Part model, mm, in its own coordinate system. A direction names the side the tool comes from. Round coordinates to 2 decimals unless told otherwise and drop trailing zeros. Loops run counter-clockwise (first coordinate to the right, second up) from the corner with the lowest first, then second, coordinate; pieces in that order, holes last. Notation, with made-up numbers: M 22.25,40 L 30.25,40 A5 ccw 30.25,48 Z; hole C -14,-37.5 d11. An arc over 180 degrees is marked long. Answer as CSV lines item,"result". Start each with the question number.
Item 1: Band-saw the part on C-C (y = -1.5). Give the cut face in (x, z), and give its area (3 significant figures).
Item 2: Which spindle directions (+Z, -Z, +X, -X, +Y, -Y) get a long thin tool onto all of the face, cutting with end or side? Do faces 4 (the cylindrical face through (0, 8.5, 5.6)), 5 (the cylindrical face through (-4.66, -8.85, 5.42)), 6 (the flat face through (8.3, -2.7, 11)), 7 (the cylindrical face through (2.406, 9.706, 5.423)), 8 (the cylindrical face through (-9.346, 3.558, 5.423)). Say none if no direction does.
Item 3: Wall check: line 1 (Y direction, x = 0, z = 3.75); line 2 (Z direction, x = 10.5, y = -6.5); line 3 (Y direction, x = 9.25, z = 3.25). Give the ranges that are in metal, low to high.
Item 4: Drop flat-ended pins along their axis: pin 1 Ø8 at (y, z) = (-7, -0.5) entering from -X; pin 2 Ø5 at (y, z) = (8, 8) entering from -X; pin 3 Ø3 at (x, y) = (0, 0) entering from -Z; pin 4 Ø1.5 at (x, z) = (0.5, 11) entering from +Y. Give the stop position or say it passes through.
Item 5: Band-saw the part on B-B (z = 8.5). Give the cut face in (x, y).
Item 6: Band-saw the part on A-A (x = 0). Give the cut face in (y, z), and give its area (3 significant figures).
Item 7: Band-saw the part on D-D (y = 3.5). Give the cut face in (x, z).
Item 8: Mould opens along X. For faces 1 (the flat face through (0, -3, 13)), 2 (the cylindrical face through (-8, -6, 5)), 3 (the cylindrical face through (-5.613, -6.383, 5.577)) say: pulls with the +X half, pulls with the -X half, needs draft (parallel to the pull), parting line crosses it, or undercut.
```python
from build123d import *

# Parameters (mm, degrees)
F0_R     = 10
F1_DEPTH = 11
F2_R     = 1.5
F3_DEPTH = 25
F4_R     = 12.5
F5_DEPTH = 2
F6_R     = 12.5
F7_DEPTH = 2
F8_R     = 2.55
F9_DEPTH = 15.001


with BuildPart() as f1:
    # F0 (on Top) → F1 (new body)
    with BuildSketch(Plane.XY):
        Circle(F0_R)
    extrude(amount=F1_DEPTH)

    # F2 (on face) → F3 (cut)
    with BuildSketch(Plane.XY.offset(11)):
        with Locations((0, 10)):
            Circle(F2_R)
        with Locations((-4.647232, 8.85456)):
            Circle(F2_R)
        with Locations((-8.229839, 5.680647)):
            Circle(F2_R)
        with Locations((-9.927089, 1.205367)):
            Circle(F2_R)
        with Locations((-9.350162, -3.546049)):
            Circle(F2_R)
        with Locations((-6.631227, -7.485107)):
            Circle(F2_R)
        with Locations((-2.393157, -9.709418)):
            Circle(F2_R)
        with Locations((2.393157, -9.709418)):
            Circle(F2_R)
        with Locations((6.631227, -7.485107)):
            Circle(F2_R)
        with Locations((9.350162, -3.546049)):
            Circle(F2_R)
        with Locations((9.927089, 1.205367)):
            Circle(F2_R)
        with Locations((8.229839, 5.680647)):
            Circle(F2_R)
        with Locations((4.647232, 8.85456)):
            Circle(F2_R)
    extrude(amount=-F3_DEPTH, mode=Mode.SUBTRACT)

    # F4 (on face) → F5 (join)
    with BuildSketch(Plane(origin=(0, 0, 0), x_dir=(1, 0, 0), z_dir=(0, 0, -1))):
        Circle(F4_R)
    extrude(amount=F5_DEPTH)

    # F6 (on face) → F7 (join)
    with BuildSketch(Plane.XY.offset(11)):
        Circle(F6_R)
    extrude(amount=F7_DEPTH)

    # F8 (on face) → F9 (cut, through all)
    with BuildSketch(Plane(origin=(0, 0, -2), x_dir=(1, 0, 0), z_dir=(0, 0, -1))):
        Circle(F8_R)
    extrude(amount=-F9_DEPTH, mode=Mode.SUBTRACT)


solid = f1.part
```
Answer block:
1,outline,"M -12.41,-2 L -2.06,-2 L -2.06,13 L -12.41,13 L -12.41,11 L -9.89,11 L -9.89,0 L -12.41,0 Z; M 2.06,-2 L 12.41,-2 L 12.41,0 L 9.89,0 L 9.89,11 L 12.41,11 L 12.41,13 L 2.06,13 Z"
1,area,"255 mm^2"
2,face 4,"+Y"
2,face 5,"-X, -Y"
2,face 6,"none"
2,face 7,"+X, +Y"
2,face 8,"-X, +Y"
3,line 1,"y = -10 to -2.55, 2.55 to 8.5"
3,line 2,"z = -2 to 0, 11 to 13"
3,line 3,"y = -2.05 to -0.13, 2.54 to 3.8"
4,pin 1,"stops at x = -12.13"
4,pin 2,"stops at x = -7.29"
4,pin 3,"passes through"
4,pin 4,"stops at y = 12.5"
5,outline,"M -10,-0.29 A10 ccw -9.78,-2.11 A1.5 cw -8.71,-4.9 A10 ccw -7.68,-6.41 A1.5 cw -5.44,-8.39 A10 ccw -3.82,-9.24 A1.5 cw -0.91,-9.96 A10 ccw 0.91,-9.96 A1.5 cw 3.82,-9.24 A10 ccw 5.44,-8.39 A1.5 cw 7.68,-6.41 A10 ccw 8.71,-4.9 A1.5 cw 9.78,-2.11 A10 ccw 10,-0.29 A1.5 cw 9.64,2.68 A10 ccw 8.99,4.39 A1.5 cw 7.29,6.85 A10 ccw 5.92,8.06 A1.5 cw 3.27,9.45 A10 ccw 1.5,9.89 A1.5 cw -1.5,9.89 A10 ccw -3.27,9.45 A1.5 cw -5.92,8.06 A10 ccw -7.29,6.85 A1.5 cw -8.99,4.39 A10 ccw -9.64,2.68 A1.5 cw Z; hole C 0,0 d5.1"
6,outline,"M -12.5,-2 L -2.55,-2 L -2.55,13 L -12.5,13 L -12.5,11 L -10,11 L -10,0 L -12.5,0 Z; M 2.55,-2 L 12.5,-2 L 12.5,0 L 8.5,0 L 8.5,11 L 12.5,11 L 12.5,13 L 2.55,13 Z"
6,area,"227 mm^2"
7,outline,"M -12,-2 L 12,-2 L 12,0 L 9.37,0 L 9.37,11 L 12,11 L 12,13 L -12,13 L -12,11 L -9.37,11 L -9.37,0 L -12,0 Z"
8,face 1,"needs draft"
8,face 2,"pulls with the -X half"
8,face 3,"undercut"
